Geometry: final body of the model. Coordinates: model frame, mm. A direction names the side the tool comes from. Round coordinates to 2 decimals unless told otherwise and drop trailing zeros. Write each loop counter-clockwise with the first axis right and the second up, starting at its lowest first coordinate (ties: lowest second). Pieces come first, ordered by that corner, then holes. Notation, with made-up numbers: (-37.75, 57.5) -> (12.25, 57.5) arc R28 ccw to (12.25, 96.5) -> close; hole circle Ø3 at (-26, 65). An arc over 180 degrees is marked (long way). Use one line per item in the form item = value. Start each with the question number.
1. Cut plane D-D, the plane z = 4.5. Return the cut outline in (x, y).
2. Draft query along X for faces 6 (the face through (28, 6, 1)), 7 (the face through (21, 6, 2)), 8 (the face through (31, 7, -1)). Return one class per face: pulls with the +X half, pulls with the -X half, needs draft (parallel to the pull), parting line crosses it, or undercut.
3. Line query: L1, parallel to Y at x = 2, z = -1.05; L2, parallel to Z at x = 18.5, y = 7; L3, parallel to Z at x = 6, y = 8. Output: solid intervals per line, ascending.
4. Cut plane C-C, the plane x = 12.5. Return the cut outline in (y, z), plus the area to 3 significant figures.
5. Pin query (flat end, axial travel): pin 1 Ø1.6 at (y, z) = (4, 1) entering from -X; pin 2 Ø5 at (x, y) = (31, 6) entering from -Z; pin 3 Ø1.5 at (x, y) = (3, 7) entering from +Z; pin 4 Ø1.2 at (x, y) = (2, 6) entering from +Z. Return the tip coordinate at first contact, or that it passes through.
6. Cut plane B-B, the plane y = 10.25. Return the cut outline in (x, z), plus the area to 3 significant figures.
7. Reachability of faces 1 (the face through (28, 6, -12)), 2 (the face through (4, 6, 0)), 3 (the face through (6, 11, 2)), 4 (the face through (4, 6, -2.5)), 5 (the face through (6, 1, 2)) from +Z, -Z, +X, -X, +Y, -Y: full face, straight path, thin tool, end or side. Return the list, or none.
8. Cut plane A-A, the plane x = 2. Return the cut outline in (y, z), plus the area to 3 significant figures.
```python
from build123d import *

# Parameters (mm, degrees)
F0_W     = 4.5
F0_H     = 12
F0_R     = 1
F0_R_2   = 2.5
F1_DEPTH = 2.5
F2_DEPTH = 2
F3_DEPTH = 22.5
F4_R     = 2.5
F5_DEPTH = 3.5
F6_DEPTH = 6.5
F8_W     = 23
F8_H     = 12
F9_DEPTH = 20


with BuildPart() as f1:
    # F0 (on Top) → F1 (new body)
    with BuildSketch(Plane.XY):
        with Locations((30.25, 6)):
            Rectangle(F0_W, F0_H)
        with Locations((31, 6)):
            Circle(F0_R, mode=Mode.SUBTRACT)
        with BuildLine():
            ThreePointArc((17, 6), (15.2426406871, 1.7573593129), (11, 0))
            Line((11, 0), (28, 0))
            Line((28, 0), (28, 12))
            Line((28, 12), (11, 12))
            ThreePointArc((11, 12), (15.2426406871, 10.2426406871), (17, 6))
        make_face()
        with BuildLine():
            Line((5, 12), (5, 6))
            ThreePointArc((5, 6), (6.7573593129, 10.2426406871), (11, 12))
            Line((11, 12), (5, 12))
        make_face()
        with BuildLine():
            Line((5, 6), (5, 0))
            Line((5, 0), (11, 0))
            ThreePointArc((11, 0), (6.7573593129, 1.7573593129), (5, 6))
        make_face()
        Polygon((0, 12), (0, 0), (5, 0), (5, 6), (5, 12), align=None)
        with Locations((2, 6)):
            Circle(F0_R, mode=Mode.SUBTRACT)
        with BuildLine():
            ThreePointArc((5, 6), (6.7573593129, 1.7573593129), (11, 0))
            ThreePointArc((11, 0), (15.2426406871, 1.7573593129), (17, 6))
            ThreePointArc((17, 6), (15.2426406871, 10.2426406871), (11, 12))
            ThreePointArc((11, 12), (6.7573593129, 10.2426406871), (5, 6))
        make_face()
        with Locations((11, 6)):
            Circle(F0_R_2, mode=Mode.SUBTRACT)
        with Locations((11, 6)):
            Circle(F0_R_2)
    extrude(amount=-F1_DEPTH)

    # F0 (on Top) → F2 (join)
    with BuildSketch(Plane.XY):
        with BuildLine():
            ThreePointArc((17, 6), (15.2426406871, 1.7573593129), (11, 0))
            Line((11, 0), (28, 0))
            Line((28, 0), (28, 12))
            Line((28, 12), (11, 12))
            ThreePointArc((11, 12), (15.2426406871, 10.2426406871), (17, 6))
        make_face()
        with BuildLine():
            Line((5, 12), (5, 6))
            ThreePointArc((5, 6), (6.7573593129, 10.2426406871), (11, 12))
            Line((11, 12), (5, 12))
        make_face()
        with BuildLine():
            Line((5, 6), (5, 0))
            Line((5, 0), (11, 0))
            ThreePointArc((11, 0), (6.7573593129, 1.7573593129), (5, 6))
        make_face()
        with BuildLine():
            ThreePointArc((5, 6), (6.7573593129, 1.7573593129), (11, 0))
            ThreePointArc((11, 0), (15.2426406871, 1.7573593129), (17, 6))
            ThreePointArc((17, 6), (15.2426406871, 10.2426406871), (11, 12))
            ThreePointArc((11, 12), (6.7573593129, 10.2426406871), (5, 6))
        make_face()
        with Locations((11, 6)):
            Circle(F0_R_2, mode=Mode.SUBTRACT)
        with Locations((11, 6)):
            Circle(F0_R_2)
    extrude(amount=F2_DEPTH)

    # F4 (on face) → F5 (join)
    with BuildSketch(Plane.XY.offset(2)):
        with BuildLine():
            ThreePointArc((11, 0), (15.2426406871, 1.7573593129), (17, 6))
            ThreePointArc((17, 6), (15.2426406871, 10.2426406871), (11, 12))
            ThreePointArc((11, 12), (6.7573593129, 10.2426406871), (5, 6))
            ThreePointArc((5, 6), (6.7573593129, 1.7573593129), (11, 0))
        make_face()
        with Locations((11, 6)):
            Circle(F4_R, mode=Mode.SUBTRACT)
    extrude(amount=F5_DEPTH)

    # F6 (add): a face of the model
    f6_faces = [f1.faces().sort_by_distance(p)[0] for p in [
        (11, 6, 2),
    ]]
    extrude(f6_faces, amount=F6_DEPTH)

    # F8 (on face) → F9 (join)
    with BuildSketch(Plane(origin=(0, 0, -2.5), x_dir=(1, 0, 0), z_dir=(0, 0, -1))):
        with Locations((16.5, -6)):
            Rectangle(F8_W, F8_H)
    extrude(amount=F9_DEPTH)


with BuildPart() as f3:
    # F0 (on Top) → F3 (new body)
    with BuildSketch(Plane.XY):
        with BuildLine():
            ThreePointArc((17, 6), (15.2426406871, 1.7573593129), (11, 0))
            Line((11, 0), (28, 0))
            Line((28, 0), (28, 12))
            Line((28, 12), (11, 12))
            ThreePointArc((11, 12), (15.2426406871, 10.2426406871), (17, 6))
        make_face()
        with BuildLine():
            ThreePointArc((5, 6), (6.7573593129, 1.7573593129), (11, 0))
            ThreePointArc((11, 0), (15.2426406871, 1.7573593129), (17, 6))
            ThreePointArc((17, 6), (15.2426406871, 10.2426406871), (11, 12))
            ThreePointArc((11, 12), (6.7573593129, 10.2426406871), (5, 6))
        make_face()
        with Locations((11, 6)):
            Circle(F0_R_2, mode=Mode.SUBTRACT)
        with Locations((11, 6)):
            Circle(F0_R_2)
        with BuildLine():
            Line((5, 12), (5, 6))
            ThreePointArc((5, 6), (6.7573593129, 10.2426406871), (11, 12))
            Line((11, 12), (5, 12))
        make_face()
        with BuildLine():
            Line((5, 6), (5, 0))
            Line((5, 0), (11, 0))
            ThreePointArc((11, 0), (6.7573593129, 1.7573593129), (5, 6))
        make_face()
    extrude(amount=-F3_DEPTH)


solid = f1.part
```
Outcome:
q1.outline = circle Ø12 at (11, 6)
q2.face_6 = pulls with the +X half
q2.face_7 = needs draft
q2.face_8 = undercut
q3.L1 = 0 to 5, 7 to 12
q3.L2 = -22.5 to 2
q3.L3 = -22.5 to 5.5
q4.outline = (0, -22.5) -> (12, -22.5) -> (12, 2) -> (11.81, 2) -> (11.81, 5.5) -> (8, 5.5) -> (8, 8.5) -> (4, 8.5) -> (4, 5.5) -> (0.19, 5.5) -> (0.19, 2) -> (0, 2) -> close
q4.area = 347 mm^2
q5.pin_1 = 5
q5.pin_2 = -2.5
q5.pin_3 = 0
q5.pin_4 = through
q6.outline = (0, -2.5) -> (5, -2.5) -> (5, -22.5) -> (28, -22.5) -> (28, -2.5) -> (32.5, -2.5) -> (32.5, 0) -> (28, 0) -> (28, 2) -> (15.24, 2) -> (15.24, 5.5) -> (6.76, 5.5) -> (6.76, 2) -> (5, 2) -> (5, 0) -> (0, 0) -> close
q6.area = 617 mm^2
q7.face_1 = -Z, +X, +Y, -Y
q7.face_2 = +Z, -X, +Y, -Y
q7.face_3 = +Z, -X, +Y
q7.face_4 = -Z, -X, +Y, -Y
q7.face_5 = +Z, -X, -Y
q8.outline = (0, -2.5) -> (5, -2.5) -> (5, 0) -> (0, 0) -> close; (7, -2.5) -> (12, -2.5) -> (12, 0) -> (7, 0) -> close
q8.area = 25.0 mm^2
